```python
from build123d import *

# Parameters (mm, degrees)
BOSS_EXTRUDE1_DEPTH = 3
SKETCH2_R           = 1.2
CUT_EXTRUDE1_DEPTH  = 105.977521403
CUT_EXTRUDE2_DEPTH  = 105.977521403


with BuildPart() as part:
    # Sketch1 → Boss-Extrude1 (new body)
    with BuildSketch(Plane(origin=(0, 0, 0), x_dir=(1, 0, 0), z_dir=(0, 1, 0))):
        with BuildLine():
            Line((-30.029977361, -66.512867647), (30.029977361, -66.512867647))
            ThreePointArc((30.029977361, -66.512867647), (32.931413623, -66.147401939), (35.651589123, -65.073836471))
            ThreePointArc((35.651589123, -65.073836471), (0, 74.2), (-35.651589123, -65.073836471))
            ThreePointArc((-35.651589123, -65.073836471), (-32.931413623, -66.147401939), (-30.029977361, -66.512867647))
        make_face()
    extrude(amount=BOSS_EXTRUDE1_DEPTH)

    # Sketch2 → Cut-Extrude1 (cut, through all)
    with BuildSketch(Plane(origin=(0, 3, 0), x_dir=(1, 0, 0), z_dir=(0, 1, 0))):
        with Locations(Location((-2.660782629, -60.941941516, 0), (0, 0, 270))):
            Circle(SKETCH2_R)
        with Locations(Location((-67.935279068, 2.966118341, 0), (0, 0, 270))):
            Circle(SKETCH2_R)
        with Locations(Location((2.922498953, 66.936230846, 0), (0, 0, 270))):
            Circle(SKETCH2_R)
        with Locations(Location((67.935279068, -2.966118341, 0), (0, 0, 270))):
            Circle(SKETCH2_R)
    extrude(amount=-CUT_EXTRUDE1_DEPTH, mode=Mode.SUBTRACT)

    # Sketch3 → Cut-Extrude2 (cut, through all)
    with BuildSketch(Plane(origin=(0, 3, 0), x_dir=(1, 0, 0), z_dir=(0, 1, 0))):
        with BuildLine():
            ThreePointArc((-74.129378041, 3.236558543), (-65.111947644, -2.5537367), (-64.529371908, 8.146832232))
            ThreePointArc((-64.529371908, 8.146832232), (-66.395420161, 10.395433666), (-66.686059299, 13.302988203))
            ThreePointArc((-66.686059299, 13.302988203), (-59.961788445, 32.071543875), (-48.083261121, 48.083261121))
            ThreePointArc((-48.083261121, 48.083261121), (-45.961940777, 48.083261121), (-45.961940777, 45.961940777))
            ThreePointArc((-45.961940777, 45.961940777), (-56.839700689, 31.531705085), (-63.324224445, 14.664330822))
            ThreePointArc((-63.324224445, 14.664330822), (-63.220830412, 12.029973663), (-61.791915049, 9.814408532))
            ThreePointArc((-61.791915049, 9.814408532), (-61.096295148, -3.187604024), (-74.099345682, -3.86354364))
            ThreePointArc((-74.099345682, -3.86354364), (-74.19933623, -0.313851977), (-74.129378041, 3.236558543))
        make_face()
        with BuildLine():
            ThreePointArc((74.129378041, -3.236558543), (65.111947644, 2.5537367), (64.529371908, -8.146832232))
            ThreePointArc((64.529371908, -8.146832232), (66.395420161, -10.395433666), (66.686059299, -13.302988203))
            ThreePointArc((66.686059299, -13.302988203), (59.961788445, -32.071543875), (48.083261121, -48.083261121))
            ThreePointArc((48.083261121, -48.083261121), (45.961940777, -48.083261121), (45.961940777, -45.961940777))
            ThreePointArc((45.961940777, -45.961940777), (56.839700689, -31.531705085), (63.324224445, -14.664330822))
            ThreePointArc((63.324224445, -14.664330822), (63.220830412, -12.029973663), (61.791915049, -9.814408532))
            ThreePointArc((61.791915049, -9.814408532), (61.096295148, 3.187604024), (74.099345682, 3.86354364))
            ThreePointArc((74.099345682, 3.86354364), (74.19933623, 0.313851977), (74.129378041, -3.236558543))
        make_face()
    extrude(amount=-CUT_EXTRUDE2_DEPTH, mode=Mode.SUBTRACT)


solid = part.part
```
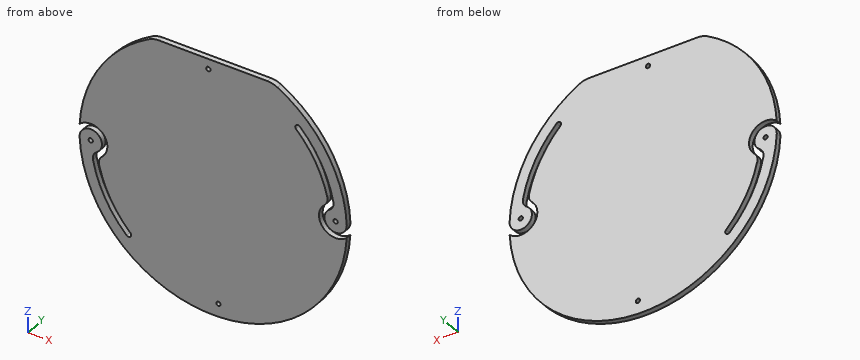
Read the model definition and answer for the solid it produces. Units are mm, in the model's axes. Give positions to 0.01 mm unless a question says otherwise; leave off trailing zeros. Loops run counter-clockwise (first coordinate to the right, second up) from the corner with the lowest first, then second, coordinate; pieces in that order, holes last.
Item 1: The part is cut by section B-B (y = 2.35). Write down the section's boundary in (x, z), and give its area (3 significant figures).
Item 2: The part is cut by section C-C (z = 0). Write down the section's boundary in (x, y), and give its area (3 significant figures).
Item 3: This flat-tipped pin is pushed along its axis until it touches: pin 1 Ø1.9 at (x, z) = (2.92, -66.94) entering from -Y. Where does it stop, or does it pass through?
Item 4: The part is cut by section A-A (x = 54.5). Write down the section's boundary in (y, z), and give its area (3 significant figures).
Item 5: Find the intervals of material crossed by line 1 along X through (y, z) = (2, -5); line 2 along Z through (x, y) = (3, 0.75); line 3 along X through (y, z) = (2.6, 2), in increasing order.
Item 6: The part is cut by section D-D (x = -53). Write down the section's boundary in (y, z).
Taken from the geometry:
1. outline: (-74.13, -3.24) arc R74.2 ccw to (74.1, -3.86) arc R9.2 cw to (61.79, 9.81) arc R5 ccw to (63.32, 14.66) arc R65 ccw to (45.96, 45.96) arc R1.5 cw to (48.08, 48.08) arc R68 cw to (66.69, 13.3) arc R5 cw to (64.53, 8.15) arc R6.2 ccw (long way) to (74.13, 3.24) arc R74.2 ccw to (35.65, 65.07) arc R11.7 ccw to (30.03, 66.51) - (-30.03, 66.51) arc R11.7 ccw to (-35.65, 65.07) arc R74.2 ccw to (-74.1, 3.86) arc R9.2 cw to (-61.79, -9.81) arc R5 ccw to (-63.32, -14.66) arc R65 ccw to (-45.96, -45.96) arc R1.5 cw to (-48.08, -48.08) arc R68 cw to (-66.69, -13.3) arc R5 cw to (-64.53, -8.15) arc R6.2 ccw (long way) to start; hole circle Ø2.4 at (-67.94, -2.97); hole circle Ø2.4 at (-2.66, 60.94); hole circle Ø2.4 at (2.92, -66.94); hole circle Ø2.4 at (67.94, 2.97)
1. area: 16,500 mm2
2. outline: (-73.38, 0) - (-62.49, 0) - (-62.49, 3) - (-73.38, 3) - close; (-59.23, 0) - (59.23, 0) - (59.23, 3) - (-59.23, 3) - close; (62.49, 0) - (73.38, 0) - (73.38, 3) - (62.49, 3) - close
2. area: 421 mm2
3. pin 1: passes through
4. outline: (0, -50.35) - (3, -50.35) - (3, 35.42) - (0, 35.42) - close; (0, 40.67) - (3, 40.67) - (3, 50.35) - (0, 50.35) - close
4. area: 286 mm2
5. line 1: x = -74.03 to -62.08, -58.96 to 63.33, 72.54 to 74.03
5. line 2: z = -74.14 to -68.13, -65.74 to 66.51
5. line 3: x = -71.65 to -64.22, -60.19 to 58.79, 61.81 to 67.22, 68.65 to 74.06
6. outline: (0, -51.93) - (3, -51.93) - (3, -42.6) - (0, -42.6) - close; (0, -37.63) - (3, -37.63) - (3, 51.93) - (0, 51.93) - close
